Check sheet for the modelled part. Datum: model origin and axes. Units: mm. A direction names the side the tool comes from. Give positions to 0.01 mm unless a question says otherwise; leave off trailing zeros. Loops run counter-clockwise (first coordinate to the right, second up) from the corner with the lowest first, then second, coordinate; pieces in that order, holes last. Notation, with made-up numbers: (66, -36.75) -> (109, -36.75) arc R31 ccw to (109, -4.75) -> close; hole circle Ø10 at (-4, -30.75). An arc over 180 degrees is marked (long way). Write each question's results on one line, items separated by ' | '. Start each with the question number.
1. Mould release check, pull along Z, two halves, no side actions. Record for faces 4 (the face through (-193.35, 131.306, 3.536)), 5 (the face through (-195.63, 128.32, 6)), 6 (the face through (-198.3, 123.9, 11.5)): +Z half, -Z half, draft (parallel to the pull), parting line (faces both ways), or undercut.
2. Material ranges on L1, parallel to X at y = 128, z = 4.5; L2, parallel to X at y = 124, z = 1.75; L3, parallel to Y at x = -198.25, z = 10.25, recorded low to high. Write a range as from..to.
3. Cross-section at B-B on x = -196.5. Record the boundary of the cut face in (y, z), and give its area (3 significant figures).
4. Cross-section at A-A on y = 125.75. Record the boundary of the cut face in (x, z) (1 decimal), and give its area (3 significant figures).
5. Cross-section at D-D on x = -195.5. Record the boundary of the cut face in (y, z), and give its area (3 significant figures).
6. Cross-section at C-C on z = 2. Record the boundary of the cut face in (x, y), and give its area (3 significant figures).
7. Gauge pin test, flat ends, axial feed: pin 1 Ø2 at (y, z) = (125.5, 6) entering from +X; pin 2 Ø1.5 at (x, y) = (-196.5, 130.5) entering from +Z (3 decimals); pin 3 Ø1 at (y, z) = (130, 4.5) entering from -X; pin 4 Ø0.5 at (x, y) = (-198, 124) entering from -Z. Record the tip position at first contact, or that the pin passes through.
8. Tool access check on faces 1 (the face through (-193.336, 131.328, 8.325)), 2 (the face through (-198.2, 124, 0.5)), 3 (the face through (-195.21, 128.05, 6)). Record the directions out of +Z, -Z, +X, -X, +Y, -Y that give a thin tool (end or side, any length) a straight path to the whole face; none if there is none.
from build123d import *

# Parameters (mm, degrees)
BOX229_W                  = 0.5
BOX229_H                  = 1
BOX229_DEPTH              = 15
BOX229_ROLL_ANGLE         = 46
BOX230_W                  = 0.5
BOX230_H                  = 1
BOX230_DEPTH              = 15
BOX230_ROLL_ANGLE         = -46
BOX227_W                  = 0.5
BOX227_H                  = 1
BOX227_DEPTH              = 11
FUSION019_PLACEMENT_ANGLE = -33.6


with BuildPart() as cubo229:
    # Box229 → Box229 (new body)
    with BuildSketch(Plane.XY):
        with Locations((0.25, 0.5)):
            Rectangle(BOX229_W, BOX229_H)
    extrude(amount=BOX229_DEPTH)


with BuildPart() as cubo229_1:
    # Box229 roll: moved
    add(cubo229.part.rotate(Axis((0, 0, 0), (1, 0, 0)), BOX229_ROLL_ANGLE))


with BuildPart() as cubo229_2:
    # Box229 placement: moved
    add(cubo229_1.part.moved(Location((0, 11, 0.5))))


with BuildPart() as cubo230:
    # Box230 → Box230 (new body)
    with BuildSketch(Plane.XY):
        with Locations((0.25, 0.5)):
            Rectangle(BOX230_W, BOX230_H)
    extrude(amount=BOX230_DEPTH)


with BuildPart() as cubo230_1:
    # Box230 roll: moved
    add(cubo230.part.rotate(Axis((0, 0, 0), (1, 0, 0)), BOX230_ROLL_ANGLE))


with BuildPart() as cubo230_2:
    # Box230 placement: moved
    add(cubo230_1.part.moved(Location((0, 0.4, 1.1))))


with BuildPart() as fusion019:
    # Box227 → Box227 (new body)
    with BuildSketch(Plane.XY.offset(0.5)):
        with Locations((0.25, 0.5)):
            Rectangle(BOX227_W, BOX227_H)
    extrude(amount=BOX227_DEPTH)

    # Fusion019: union Cubo229, Cubo230
    add(cubo229_2.part)
    add(cubo230_2.part)


with BuildPart() as fusion019_1:
    # Fusion019 placement: moved
    add(fusion019.part.moved(Location((-198.7, 123.7, 0))).rotate(Axis((-198.7, 123.7, 0), (0, 0, 1)), FUSION019_PLACEMENT_ANGLE))


solid = fusion019_1.part
Geometry says:
1) face 4: undercut | face 5: draft | face 6: +Z half
2) L1: -195.84..-195.49 | L2: -198.5..-197.9 | L3: 123.47..124.38
3) outline: (126.11, 2.44) -> (127.01, 3.16) -> (127.01, 4.55) -> (126.11, 3.83) -> close; (126.11, 8.01) -> (127.01, 7.28) -> (127.01, 8.67) -> (126.11, 9.4) -> close | area: 2.51 mm^2
4) outline: (-197.3, 1.7) -> (-196.7, 2) -> (-196.7, 3.4) -> (-197.3, 3.1) -> close; (-197.3, 8.7) -> (-196.7, 8.4) -> (-196.7, 9.8) -> (-197.3, 10.1) -> close | area: 1.67 mm^2
5) outline: (127.61, 4.18) -> (128.52, 4.91) -> (128.52, 6.93) -> (127.61, 7.66) -> (127.61, 6.27) -> (128.04, 5.92) -> (127.61, 5.57) -> close | area: 2.33 mm^2
6) outline: (-198.7, 123.7) -> (-198.28, 123.42) -> (-197.73, 124.26) -> (-198.15, 124.53) -> close; (-197.96, 124.81) -> (-197.55, 124.53) -> (-196.75, 125.73) -> (-197.17, 126.01) -> close; (-193.47, 131.57) -> (-193.06, 131.29) -> (-192.26, 132.49) -> (-192.68, 132.77) -> close | area: 1.94 mm^2
7) pin 1: x = -198.1 | pin 2: through | pin 3: x = -194.85 | pin 4: z = 0.5
8) face 1: +X, +Y | face 2: -Z, -X, -Y | face 3: +Z, -Z, +X, -Y
